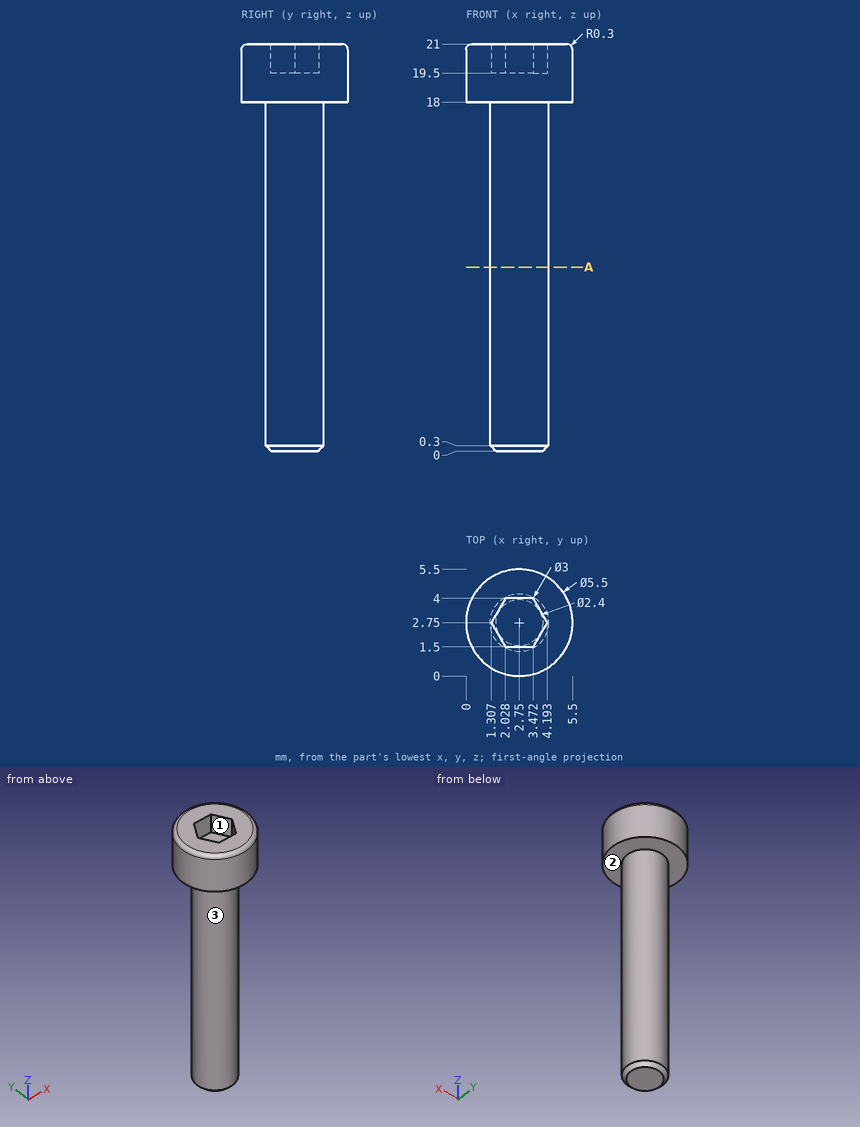
Could you check a few things on this drawing? It's one solid part, dimensions in mm from its lowest x, y, z. Give positions to 0.01 mm unless a question says otherwise; leave off trailing zeros. Loops run counter-clockwise (first coordinate to the right, second up) from the corner with the lowest first, then second, coordinate; pieces in that order, holes last. Notation, with made-up numbers: M 19.25,21 L 75.25,21 A20 ccw 75.25,38 Z; hole C -23,49 d7. An arc over 180 degrees is marked long. Return JSON: item names as keys, results as strings.
Item 1: Imagine slicing it at A-A on z = 9.5. List the corners of the cut face in (x, y) for me.
A:
{"outline": "C 2.75,2.75 d3"}
Item 2: I'm going to push flat-ended pins straight in: pin 1 Ø1 at (x, z) = (4.5, 12) entering from -Y; pin 2 Ø1.2 at (x, y) = (2.5, 2.5) entering from +Z; pin 3 Ø1.5 at (y, z) = (3, 3.5) entering from -X. Where does each tip first touch, or does it pass through?
A:
{"pin 1": "stops at y = 1.92", "pin 2": "stops at z = 19.5", "pin 3": "stops at x = 1.25"}
Item 3: Please list where these lines run through material, in increasing order: line 1 (Y direction, x = 2.7, z = 4.5); line 2 (Z direction, x = 2.4, y = 2.85); line 3 (Z direction, x = 4.4, y = 3.85).
A:
{"line 1": "y = 1.25 to 4.25", "line 2": "z = 0 to 19.5", "line 3": "z = 18 to 21"}
Item 4: Thinking about a two-plate mould opening in X: for the marked faces 1, 2 and 3, which applies, released by +X, released by -X, zero draft, split by the parting line, or undercut?
A:
{"face 1": "undercut", "face 2": "zero draft", "face 3": "split by the parting line"}
